from build123d import *

# Parameters (mm, degrees)
BOSS_EXTRUDE1_DEPTH      = 76.2
BOSS_EXTRUDE1_DEPTH_BACK = 76.2
M12_CLEARANCE_HOLE1_D    = 13.5
F_1_2_CLEARANCE_HOLE1_D  = 13.49248


with BuildPart() as part:
    # Sketch3 → Boss-Extrude1 (new, two sides: drawn at the far end of the back side and taken through both)
    with BuildSketch(Plane.XY.offset(-BOSS_EXTRUDE1_DEPTH_BACK)):
        with BuildLine():
            Line((0, 19.05), (0, 83.82))
            ThreePointArc((0, 83.82), (-1.487897552, 87.412102448), (-5.08, 88.9))
            Line((-5.08, 88.9), (-12.7, 88.9))
            Line((-12.7, 88.9), (-12.7, -12.7))
            Line((-12.7, -12.7), (88.9, -12.7))
            Line((88.9, -12.7), (88.9, -5.08))
            ThreePointArc((88.9, -5.08), (87.412102448, -1.487897552), (83.82, 0))
            Line((83.82, 0), (19.05, 0))
            ThreePointArc((19.05, 0), (5.579615818, 5.579615818), (0, 19.05))
        make_face()
    extrude(amount=BOSS_EXTRUDE1_DEPTH + BOSS_EXTRUDE1_DEPTH_BACK)

    # M12 Clearance Hole1 (through all)
    with Locations(Plane(origin=(0, 0, 0), x_dir=(0, 0, -1), z_dir=(1, 0, 0))):
        with Locations((0, 38.1)):
            Hole(M12_CLEARANCE_HOLE1_D / 2)

    # 1/2 Clearance Hole1 (through all)
    with Locations(Plane(origin=(0, 0, 0), x_dir=(1, 0, 0), z_dir=(0, 1, 0))):
        with Locations((51.435, -45.72), (51.435, 45.72), (51.435, 15.24), (51.435, -15.24)):
            Hole(F_1_2_CLEARANCE_HOLE1_D / 2)


solid = part.part
CAD build for the part. Positions are in the model's coordinates, mm. A direction names the side the tool comes from. Give positions to 0.01 mm unless a question says otherwise; leave off trailing zeros. Write each loop counter-clockwise with the first axis right and the second up, starting at its lowest first coordinate (ties: lowest second). Pieces come first, ordered by that corner, then holes. Notation, with made-up numbers: (42.5, 12.25) - (69.5, 12.25) arc R25 ccw to (69.5, 40.25) - close; hole circle Ø5 at (-12, 5.5). An arc over 180 degrees is marked (long way). Answer as CSV lines item,"result".
Q1. Pull direction X, two halves, no side cores. Call faces 3 (the face through (87.451, -1.528, -1.067)), 4 (the face through (-12.7, 50, -1)), 5 (the face through (56.79, -6.44, -11.14)): released by +X, released by -X, zero draft, split by the parting line, or undercut.
Result set:
face 3,"released by +X"
face 4,"released by -X"
face 5,"undercut"
Q2. 3-axis set-ups, long thin cutter, end or side, ignore diameter. For faces 1 (the face through (52, 0, -1)), 2 (the face through (-6.44, 32.11, 3.11)): which of +Z, -Z, +X, -X, +Y, -Y reach the whole face in a straight line?
Result set:
face 1,"+Z, -Z, +X, +Y"
face 2,"+X, -X"
Q3. Band-saw the part on C-C (z = -61). Give the cut face in (x, y).
Result set:
outline,"(-12.7, -12.7) - (88.9, -12.7) - (88.9, -5.08) arc R5.08 ccw to (83.82, 0) - (19.05, 0) arc R19.05 cw to (0, 19.05) - (0, 83.82) arc R5.08 ccw to (-5.08, 88.9) - (-12.7, 88.9) - close"
Q4. Band-saw the part on D-D (x = 55.5). Give the cut face in (y, z), and give its area (3 significant figures).
Result set:
outline,"(-12.7, -76.2) - (0, -76.2) - (0, -51.1) - (-12.7, -51.1) - close; (-12.7, -40.34) - (0, -40.34) - (0, -20.62) - (-12.7, -20.62) - close; (-12.7, -9.86) - (0, -9.86) - (0, 9.86) - (-12.7, 9.86) - close; (-12.7, 20.62) - (0, 20.62) - (0, 40.34) - (-12.7, 40.34) - close; (-12.7, 51.1) - (0, 51.1) - (0, 76.2) - (-12.7, 76.2) - close"
area,"1,390 mm²"
Q5. Band-saw the part on B-B (y = -3). Give the cut face in (x, z) (3 decimals).
Result set:
outline,"(-12.7, -76.2) - (88.455, -76.2) - (88.455, 76.2) - (-12.7, 76.2) - close; hole circle Ø13.492 at (51.435, -45.72); hole circle Ø13.492 at (51.435, -15.24); hole circle Ø13.492 at (51.435, 15.24); hole circle Ø13.492 at (51.435, 45.72)"
Q6. Band-saw the part on A-A (z = 0). Give the cut face in (x, y).
Result set:
outline,"(-12.7, -12.7) - (88.9, -12.7) - (88.9, -5.08) arc R5.08 ccw to (83.82, 0) - (19.05, 0) arc R19.05 cw to (0, 19.05) - (0, 31.35) - (-12.7, 31.35) - close; (-12.7, 44.85) - (0, 44.85) - (0, 83.82) arc R5.08 ccw to (-5.08, 88.9) - (-12.7, 88.9) - close"
Q7. Drill centre lines: line 1 (Y direction, x = -5, z = 0); line 2 (Y direction, x = 59, z = -28); line 3 (X direction, y = -9, z = -15). Where is each one in solid material? Low to high. Write a range as from..to.
Result set:
line 1,"-12.7..31.35, 44.85..88.9"
line 2,"-12.7..0"
line 3,"-12.7..44.69, 58.18..88.9"
Q8. Flat gauge pins, fed straight in: pin 1 Ø6 at (y, z) = (21, 53.5) entering from +X; pin 2 Ø12 at (x, z) = (62.5, -56) entering from +Y. Where does each tip first touch, or does it go through?
Result set:
pin 1,"x = 0.03"
pin 2,"y = 0"
